Could you check a few things on this model? Use its own coordinates, in mm. A direction names the side the tool comes from. Round coordinates to 2 decimals unless told otherwise and drop trailing zeros. Order: outer loops, then holes, each group sorted by start corner. A loop starts at its lowest first (then second) coordinate and runs counter-clockwise, first axis right, second up.
```python
from build123d import *

# Parameters (mm, degrees)
F0_W           = 152.4
F0_H           = 76.2
F1_DEPTH       = 25.4
F2_W           = 147.32
F2_H           = 71.12
F3_DEPTH       = 5.08
F5_DEPTH       = 2.54
F6_SIZE        = 2.53999
F8_DEPTH       = 2.54
F9_SIZE        = 2.53999
F10_W          = 64.77
F10_H          = 25.4
F10_W_2        = 5.715
F11_DEPTH      = 5.715
F11_DEPTH_BACK = 2.54


# Not quite as in the source:
# - a fillet or chamfer is up to 0.001 mm smaller than in the source, because OpenCascade refuses the exact size


with BuildPart() as f1:
    # F0 (on Top) → F1 (new body)
    with BuildSketch(Plane.XY):
        with Locations((76.2, 38.1)):
            Rectangle(F0_W, F0_H)
    extrude(amount=F1_DEPTH)

    # F2 (on face) → F3 (cut)
    with BuildSketch(Plane.XY.offset(25.4)):
        with Locations((76.2, 38.1)):
            Rectangle(F2_W, F2_H)
    extrude(amount=-F3_DEPTH, mode=Mode.SUBTRACT)

    # F4 (on face) → F5 (cut)
    with BuildSketch(Plane.XZ):
        with BuildLine():
            Line((8.89, 12.7), (8.89, 0))
            Line((8.89, 0), (143.51, 0))
            Line((143.51, 0), (143.51, 12.7))
            ThreePointArc((143.51, 12.7), (141.6501280605, 17.1901280605), (137.16, 19.05))
            Line((137.16, 19.05), (15.24, 19.05))
            ThreePointArc((15.24, 19.05), (10.7498719395, 17.1901280605), (8.89, 12.7))
        make_face()
    extrude(amount=-F5_DEPTH, mode=Mode.SUBTRACT)

    # F6 (size 2.54 in the source; OpenCascade refuses exactly that, so slightly less here)
    f6_edges = [f1.edges().sort_by_distance(p)[0] for p in [
        (76.2, 2.54, 19.05),
    ]]
    chamfer(f6_edges, length=F6_SIZE)

    # F7 (on face) → F8 (cut)
    with BuildSketch(Plane(origin=(0, 76.2, 0), x_dir=(-1, 0, 0), z_dir=(0, 1, 0))):
        with BuildLine():
            Line((-143.51, 12.7), (-143.51, 0))
            Line((-143.51, 0), (-8.89, 0))
            Line((-8.89, 0), (-8.89, 12.7))
            ThreePointArc((-8.89, 12.7), (-10.7498719395, 17.1901280605), (-15.24, 19.05))
            Line((-15.24, 19.05), (-137.16, 19.05))
            ThreePointArc((-137.16, 19.05), (-141.6501280605, 17.1901280605), (-143.51, 12.7))
        make_face()
    extrude(amount=-F8_DEPTH, mode=Mode.SUBTRACT)

    # F9 (size 2.54 in the source; OpenCascade refuses exactly that, so slightly less here)
    f9_edges = [f1.edges().sort_by_distance(p)[0] for p in [
        (76.2, 73.66, 19.05),
    ]]
    chamfer(f9_edges, length=F9_SIZE)

    # F10 (on face) → F11 (join, two sides)
    with BuildSketch(Plane.YZ.offset(152.4)) as f11_sk:
        with BuildLine():
            Line((5.715, 40.1454963986), (5.715, 25.4))
            Line((5.715, 25.4), (70.485, 25.4))
            Line((70.485, 25.4), (70.485, 40.1454963986))
            ThreePointArc((70.485, 40.1454963986), (38.1, 44.5135), (5.715, 40.1454963986))
        make_face()
        with Locations((38.1, 12.7)):
            Rectangle(F10_W, F10_H)
        with Locations((2.8575, 12.7)):
            Rectangle(F10_W_2, F10_H)
        Polygon((0, 63.5), (0, 25.4), (5.715, 25.4), (5.715, 40.1454963986), (5.715, 63.5), align=None)
        Polygon((70.485, 40.1454963986), (70.485, 25.4), (76.2, 25.4), (76.2, 63.5), (70.485, 63.5), align=None)
        with Locations((73.3425, 12.7)):
            Rectangle(F10_W_2, F10_H)
    extrude(amount=F11_DEPTH)
    extrude(f11_sk.sketch, amount=-F11_DEPTH_BACK)


solid = f1.part
```
Q1. For faces 1 (the flat face through (75, 2.54, 8)), 2 (the flat face through (154, 70.485, 52)), 3 (the conical face through (140.527, 74.666, 16.142)), which set-ups out of +Z, -Z, +X, -X, +Y, -Y let a thin tool reach every point of the face, with its end or its side?
Q2. Imagine slicing it at D-D, the plane y = 32.5. Please give me the cut outline in (x, z) (3 decimals), then the cut area to 3 significant figures.
Q3. We'd pull the mould along X, two halves only. Please class faces 4 (the flat face through (2.54, 38, 23)), 5 (the flat face through (154, 73, 63.5)), 6 (the flat face through (0, 38, 13)): released by +X, released by -X, zero draft, split by the parting line, or undercut.
Q4. Imagine slicing it at A-A, the plane z = 60. Please give me the cut outline in (x, y) (3 decimals), then the cut area to 3 significant figures.
Q5. I need wall thicknesses on L1, parallel to Z at x = 100, y = 51; L2, parallel to Y at x = 88.5, z = 23.5; L3, parallel to X at y = 34, z = 36 (3 decimals). Which ranges of each line are inside material? Lowest first, please.
Q6. For P1, Ø8.5, axis at x = 94, z = 8, coming from the -Y side; P2, Ø21.5, axis at y = 45, z = 51, coming from the -X side; P3, Ø2, axis at x = 37, z = 16, coming from the +Y side, each with a flat end and sliding along its axis, tell me the tip position at first contact or that it passes through.
Filled in:
1. face 1: -Z, -Y
1. face 2: +Z, +X, -X
1. face 3: -Z, +Y
2. outline: (0, 0) - (158.115, 0) - (158.115, 44.385) - (149.86, 44.385) - (149.86, 20.32) - (2.54, 20.32) - (2.54, 25.4) - (0, 25.4) - close
2. area: 3,420 mm2
3. face 4: undercut
3. face 5: zero draft
3. face 6: released by -X
4. outline: (149.86, 0) - (158.115, 0) - (158.115, 5.715) - (149.86, 5.715) - close; (149.86, 70.485) - (158.115, 70.485) - (158.115, 76.2) - (149.86, 76.2) - close
4. area: 94.4 mm2
5. L1: z = 0 to 20.32
5. L2: y = 0 to 2.54, 73.66 to 76.2
5. L3: x = 149.86 to 158.115
6. P1: stops at y = 2.54
6. P2: stops at x = 149.86
6. P3: stops at y = 74.15
